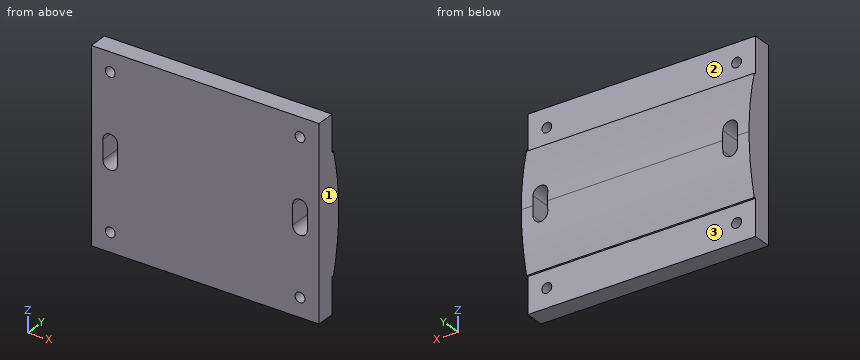
```python
from build123d import *

# Parameters (mm, degrees)
SKETCH_1_W             = 600
SKETCH_1_H             = 500
EXTRUDE_1_DEPTH        = 75
CUT_EXTRUDE_1_DEPTH    = 785.617741324
CUT_EXTRUDE_2_DEPTH    = 785.617741324
SKETCH_5_R             = 13
CUT_EXTRUDE_3_DEPTH    = 783.623792125
CUT_EXTRUDE_4_DEPTH    = 785.617741324
PATTERN_LINEAR_1_COUNT = 2
PATTERN_LINEAR_1_PITCH = 500


with BuildPart() as part:
    # 草图1 → 凸台-拉伸1 (new body)
    with BuildSketch(Plane(origin=(0, 0, 0), x_dir=(1, 0, 0), z_dir=(0, 1, 0))):
        with Locations((300, 250)):
            Rectangle(SKETCH_1_W, SKETCH_1_H)
    extrude(amount=EXTRUDE_1_DEPTH)

    # 草图3 → 切除-拉伸1 (cut, through all)
    with BuildSketch(Plane(origin=(600, 0, 0), x_dir=(0, 0, -1), z_dir=(1, 0, 0))):
        with BuildLine():
            Line((405, 55), (405, 50))
            Line((405, 50), (500, 50))
            Line((500, 50), (500, 75))
            Line((500, 75), (250, 75))
            ThreePointArc((250, 75), (328.14249804, 69.979359813), (405, 55))
        make_face()
    extrude(amount=-CUT_EXTRUDE_1_DEPTH, mode=Mode.SUBTRACT)

    # 草图4 → 切除-拉伸2 (cut, through all)
    with BuildSketch(Plane(origin=(600, 0, 0), x_dir=(0, 0, -1), z_dir=(1, 0, 0))):
        with BuildLine():
            Line((0, 75), (0, 50))
            Line((0, 50), (95, 50))
            Line((95, 50), (95, 55))
            ThreePointArc((95, 55), (171.85750196, 69.979359813), (250, 75))
            Line((250, 75), (0, 75))
        make_face()
    extrude(amount=-CUT_EXTRUDE_2_DEPTH, mode=Mode.SUBTRACT)

    # 草图5 → 切除-拉伸3 (cut, through all)
    with BuildSketch(Plane(origin=(0, 50, 0), x_dir=(1, 0, 0), z_dir=(0, 1, 0))):
        with Locations(Location((50, 450, 0), (0, 0, 270))):
            Circle(SKETCH_5_R)
        with Locations(Location((550, 450, 0), (0, 0, 270))):
            Circle(SKETCH_5_R)
        with Locations(Location((50, 50, 0), (0, 0, 270))):
            Circle(SKETCH_5_R)
        with Locations(Location((550, 50, 0), (0, 0, 270))):
            Circle(SKETCH_5_R)
    extrude(amount=-CUT_EXTRUDE_3_DEPTH, mode=Mode.SUBTRACT)

    # 草图6 → 切除-拉伸4 (cut, through all)
    with BuildSketch(Plane.XZ):
        with BuildLine():
            Line((30.5, -224.5), (30.5, -275.5))
            ThreePointArc((30.5, -275.5), (50, -295), (69.5, -275.5))
            Line((69.5, -275.5), (69.5, -224.5))
            ThreePointArc((69.5, -224.5), (50, -205), (30.5, -224.5))
        make_face()
    cut_extrude_4 = extrude(amount=-CUT_EXTRUDE_4_DEPTH, mode=Mode.SUBTRACT)

    # 阵列(线性)1: 切除-拉伸4 ×2
    with Locations(*[(i * PATTERN_LINEAR_1_PITCH, 0, 0) for i in range(1, PATTERN_LINEAR_1_COUNT)]):
        add(cut_extrude_4, mode=Mode.SUBTRACT)


solid = part.part
```
Input: part model. Units: mm. Frame: model coordinates. Face numbers are marked on the shaded views. A direction names the side the tool comes from. Coordinates: 2 decimals unless noted, no trailing zeros. Write each loop counter-clockwise with the first axis right and the second up, starting at its lowest first coordinate (ties: lowest second). Pieces come first, ordered by that corner, then holes. Notation, with made-up numbers: M 21,17.25 L 75,17.25 A32 cw 75,51.25 Z; hole C -24,32.5 d1. An arc over 180 degrees is marked long. Use one line per item in the form item = value.
Q1. Section A-A (z = -50). Return loops of the section in (x, y), plus the area to 3 significant figures.
Answer below:
outline = M 0,0 L 37,0 L 37,50 L 0,50 Z; M 63,0 L 537,0 L 537,50 L 63,50 Z; M 563,0 L 600,0 L 600,50 L 563,50 Z
area = 27,400 mm²
Q2. First-contact query: pin 1 (23.5 mm diameter, centred on x = 50, z = -450, fed in from +Y); pin 2 (2.5 mm diameter, centred on x = 385.5, y = 52.5, fed in from +Z); pin 3 (3 mm diameter, centred on x = 413, z = -168, fed in from +Y); pin 4 (2 mm diameter, centred on x = 195, z = -269, fed in from +Y). Flat tips, straight axial feed; report the tip coordinate or a pass-through.
Answer below:
pin_1 = through
pin_2 = -95
pin_3 = 69.67
pin_4 = 74.73
Q3. Set-up query: the marked faces 1, 2 and 3. Return all of +Z, -Z, +X, -X, +Y, -Y with unobstructed straight access to the full face (end or side cutting, diameter ignored); none if empty.
Answer below:
face_1 = +Z, -Z, +X, +Y, -Y
face_2 = +Z, +X, -X, +Y
face_3 = -Z, +X, -X, +Y
Q4. Material intervals for probe 1 along Z at (x, y) = (550, 40); probe 2 along X at (y, z) = (58, -271.5); probe 3 along X at (y, z) = (26, -450), sorted ascending. Write a range as from..to.
Answer below:
probe_1 = -500..-463, -437..-295, -205..-63, -37..0
probe_2 = 0..30.5, 69.5..530.5, 569.5..600
probe_3 = 0..37, 63..537, 563..600
Q5. Section C-C (y = 17.5). Return loops of the section in (x, z).
Answer below:
outline = M 0,-500 L 600,-500 L 600,0 L 0,0 Z; hole M 30.5,-275.5 A19.5 ccw 69.5,-275.5 L 69.5,-224.5 A19.5 ccw 30.5,-224.5 Z; hole C 50,-450 d26; hole C 50,-50 d26; hole M 530.5,-275.5 A19.5 ccw 569.5,-275.5 L 569.5,-224.5 A19.5 ccw 530.5,-224.5 Z; hole C 550,-450 d26; hole C 550,-50 d26
Q6. Section D-D (x = 168.5). Return loops of the section in (y, z) (3 decimals), plus the area to 3 significant figures.
Answer below:
outline = M 0,-500 L 50,-500 L 50,-405 L 55,-405 A610.625 ccw 55,-95 L 50,-95 L 50,0 L 0,0 Z
area = 30,700 mm²
Q7. Section B-B (x = 50). Return loops of the section in (y, z) (3 decimals), plus the area to 3 significant figures.
Answer below:
outline = M 0,-500 L 50,-500 L 50,-463 L 0,-463 Z; M 0,-437 L 50,-437 L 50,-405 L 55,-405 A610.625 ccw 73.34,-295 L 0,-295 Z; M 0,-205 L 73.34,-205 A610.625 ccw 55,-95 L 50,-95 L 50,-63 L 0,-63 Z; M 0,-37 L 50,-37 L 50,0 L 0,0 Z
area = 21,400 mm²
